Read the model definition and answer for the solid it produces. Units are mm, in the model's axes. Face numbers are marked on the shaded views. A direction names the side the tool comes from. Coordinates: 2 decimals unless noted, no trailing zeros. Order: outer loops, then holes, each group sorted by start corner. A loop starts at its lowest first (then second) coordinate and runs counter-clockwise, first axis right, second up. Notation, with made-up numbers: (60.25, 42) -> (103.25, 42) arc R28 cw to (103.25, 70) -> close; hole circle Ø1 at (76.25, 11.5). An arc over 180 degrees is marked (long way). Return JSON: item names as keys, results as strings. Group by question number.
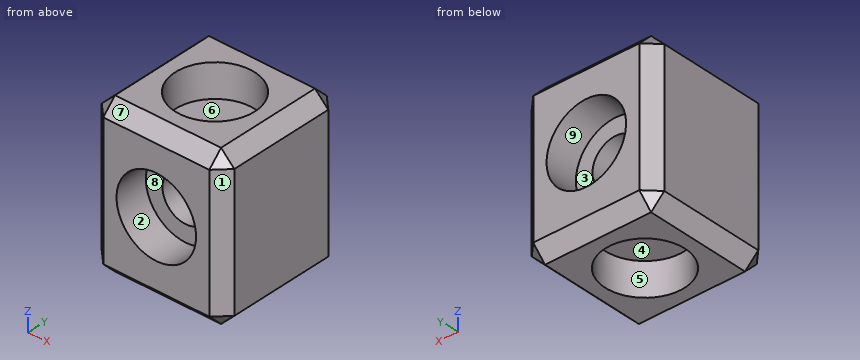
Autodesk Inventor part; units mm, degrees
ref_plane "YZ Plane" through (0, 0, 0) normal (1, 0, 0) x (0, 1, 0)
ref_plane "XZ Plane" through (0, 0, 0) normal (0, 1, 0) x (-1, 0, 0)
ref_plane "XY Plane" through (0, 0, 0) normal (0, 0, 1) x (1, 0, 0)
sketch "Esquisse1" plane through (0, 0, 0) normal (0, 1, 0) x (-1, 0, 0)
  line L0 (5, 6) -> (-5, 6)
  line L1 (-5, 6) -> (-5, -6)
  line L2 (-5, -6) -> (5, -6)
  line L3 (5, -6) -> (5, 6)
  point P0 (0, 0)
  dimension "d0" = 10
  dimension "d1" = 5
  dimension "d2" = 6
  dimension "d3" = 6
extrude "Extrusion1" add sketch "Esquisse1" along normal blind 10
sketch "Esquisse2" plane through (-5, 0, 6) normal (0, 0, 1) x (1, 0, 0)
  circle A0 centre (5, 5) radius 3
  line L0 (0, 0) -> (0, 10)
  point P0 (5, 0)
  dimension "d6" = 6
  dimension "d7" = 5
  dimension "d8" = 5
extrude "Extrusion2" cut sketch "Esquisse2" against normal blind 2.5
sketch "Esquisse3" plane through (5, 0, -6) normal (0, 0, -1) x (-1, 0, 0)
  circle A0 centre (5, 5) radius 3
  point P0 (5, 0)
extrude "Extrusion3" cut sketch "Esquisse3" against normal blind 2.5
sketch "Esquisse4" plane through (0, 0, 0) normal (0, -1, 0) x (1, 0, 0)
  circle A0 centre (0, 0) radius 3
  dimension "d13" = 6
extrude "Extrusion4" cut sketch "Esquisse4" against normal blind 2.5
sketch "Esquisse5" plane through (0, 10, 0) normal (0, 1, 0) x (1, 0, 0)
  circle A0 centre (0, 0) radius 3
  circle A1 centre (0, 0) radius 3
extrude "Extrusion5" cut sketch "Esquisse5" against normal blind 2.5
sketch "Esquisse6" plane through (0, 7.5, 0) normal (0, 1, 0) x (1, 0, 0)
  circle A0 centre (0, 0) radius 1.75
  dimension "d18" = 3.5
extrude "Extrusion6" cut sketch "Esquisse6" against normal up to surface (5 mm away)
chamfer "Chanfrein1" distance 1 angle 45 12 edges at (5, 10, 0) (0, 10, 6) (5, 5, 6) (-5, 5, 6) (0, 0, 6) (5, 0, 0) (5, 5, -6) (0, 0, -6) (-5, 0, 0) (-5, 10, 0) (0, 10, -6) (-5, 5, -6)
properties part number "piece roulement"
1. Find section B-B on y = 5. Determine the outline of the cut face in (x, z), and give its area (3 significant figures).
2. Straight lines are drawn through the part: L1, parallel to X at y = 4.7, z = 0; L2, parallel to Z at x = 0, y = 8.2; L3, parallel to Z at x = 2.5, y = 4. For each, find the intervals that lie inside material, in ascending order.
3. For a pull along Y with two mould halves and no side action, classify the marked faces 1, 2, 3 and 4 as released by +Y, released by -Y, zero draft, split by the parting line, or undercut.
4. Find section C-C on z = -3.75. Determine the outline of the cut face in (x, y), and give its area (3 significant figures).
5. Find section D-D on z = 0. Determine the outline of the cut face in (x, y), and give its area (3 significant figures).
6. Find section A-A on x = 0. Determine the outline of the cut face in (y, z), and give its area (3 significant figures).
7. Given pin 1 (5 mm diameter, centred on x = 0, z = 0, fed in from +Y), flat-ended and moving along its own axis, determine where the tip first touches the part or whether it passes through.
8. Which of the six approach directions +Z, -Z, +X, -X, +Y, -Y give full straight-line access (tool end or side, diameter ignored) to the marked faces 5, 6, 7, 8 and 9?
Result:
{
 "1": {"outline": "(-5, -5) -> (-4, -6) -> (-3, -6) -> (-3, -3.5) -> (3, -3.5) -> (3, -6) -> (4, -6) -> (5, -5) -> (5, 5) -> (4, 6) -> (3, 6) -> (3, 3.5) -> (-3, 3.5) -> (-3, 6) -> (-4, 6) -> (-5, 5) -> close; hole circle Ø3.5 at (0, 0)", "area": "78.4 mm^2"},
 "2": {"L1": "-5 to -1.75, 1.75 to 5", "L2": "-6 to -3, 3 to 6", "L3": "-3.5 to 3.5"},
 "3": {"face 1": "released by -Y", "face 2": "zero draft", "face 3": "released by +Y", "face 4": "undercut"},
 "4": {"outline": "(-5, 1) -> (-4, 0) -> (4, 0) -> (5, 1) -> (5, 9) -> (4, 10) -> (-4, 10) -> (-5, 9) -> close; hole circle Ø6 at (0, 5)", "area": "69.7 mm^2"},
 "5": {"outline": "(-5, 1) -> (-4, 0) -> (-3, 0) -> (-3, 2.5) -> (-1.75, 2.5) -> (-1.75, 7.5) -> (-3, 7.5) -> (-3, 10) -> (-4, 10) -> (-5, 9) -> close; (1.75, 2.5) -> (3, 2.5) -> (3, 0) -> (4, 0) -> (5, 1) -> (5, 9) -> (4, 10) -> (3, 10) -> (3, 7.5) -> (1.75, 7.5) -> close", "area": "50.5 mm^2"},
 "6": {"outline": "(0, -5) -> (1, -6) -> (2, -6) -> (2, -3.5) -> (8, -3.5) -> (8, -6) -> (9, -6) -> (10, -5) -> (10, -3) -> (7.5, -3) -> (7.5, -1.75) -> (2.5, -1.75) -> (2.5, -3) -> (0, -3) -> close; (0, 3) -> (2.5, 3) -> (2.5, 1.75) -> (7.5, 1.75) -> (7.5, 3) -> (10, 3) -> (10, 5) -> (9, 6) -> (8, 6) -> (8, 3.5) -> (2, 3.5) -> (2, 6) -> (1, 6) -> (0, 5) -> close", "area": "40.5 mm^2"},
 "7": {"pin 1": "y = 7.5"},
 "8": {"face 5": "-Z", "face 6": "+Z", "face 7": "+Z, +X, -X, -Y", "face 8": "-Y", "face 9": "+Y"}
}
